Check sheet for the modelled part. Datum: model origin and axes. Units: mm. Coordinates: 2 decimals unless noted, no trailing zeros. Order: outer loops, then holes, each group sorted by start corner. A loop starts at its lowest first (then second) coordinate and runs counter-clockwise, first axis right, second up.
1. Draft check along Y on faces 1 (the cylindrical face through (21.09, -41.027, 1.29)), 2 (the cylindrical face through (-16.44, 33.2, 1.29)), 3 (the flat face through (0, 1, 2)), 4 (the cylindrical face through (24.837, 48.709, 1.29)). Enter one of: released by +Y, released by -Y, zero draft, split by the parting line, or undercut.
2. Thickness scan on line 1 (X direction, y = 10, z = 1.05); line 2 (Y direction, x = 21.5, z = 1.65). Record the ranges inside material, lowest first.
3. Cross-section at A-A (y = -10.5). Enter the section's corners in (x, z).
4. Gauge pin test, flat ends, axial feed: pin 1 Ø0.7 at (x, z) = (6, 1) entering from +Y; pin 2 Ø0.7 at (x, z) = (-12, 1.5) entering from +Y; pin 3 Ø1.1 at (x, z) = (8.5, 1) entering from +Y; pin 4 Ø2.5 at (x, y) = (15.25, 3.61) entering from +Z. Record the tip position at first contact, or that the pin passes through.
```python
from build123d import *

# Parameters (mm, degrees)
F0_R     = 3.15
F0_W     = 5
F0_H     = 2.5
F0_W_2   = 30
F0_H_2   = 13
F0_R_2   = 1.5
F1_DEPTH = 2
F2_SIZE  = 0.6
F3_SIZE  = 1


with BuildPart() as f1:
    # F0 (on Top) → F1 (new body)
    with BuildSketch(Plane.XY):
        with BuildLine():
            ThreePointArc((19.649657, 49.48842), (0, 46.17961), (-19.649657, 49.48842))
            ThreePointArc((-19.649657, 49.48842), (-24.776283, 48.753093), (-27.15, 44.15))
            Line((-27.15, 44.15), (-27.15, -44.15))
            ThreePointArc((-27.15, -44.15), (-24.776283, -48.753093), (-19.649657, -49.48842))
            ThreePointArc((-19.649657, -49.48842), (0, -46.17961), (19.649657, -49.48842))
            ThreePointArc((19.649657, -49.48842), (24.776283, -48.753093), (27.15, -44.15))
            Line((27.15, -44.15), (27.15, 44.15))
            ThreePointArc((27.15, 44.15), (24.776283, 48.753093), (19.649657, 49.48842))
        make_face()
        with Locations((-21.5, -44.15)):
            Circle(F0_R, mode=Mode.SUBTRACT)
        with Locations((-12.882352, -38.913459)):
            Rectangle(F0_W, F0_H, mode=Mode.SUBTRACT)
        with Locations((-12.882352, -5.600822)):
            Rectangle(F0_W, F0_H, mode=Mode.SUBTRACT)
        with Locations((7.687139, -38.913459)):
            Rectangle(F0_W, F0_H, mode=Mode.SUBTRACT)
        with Locations((21.5, -44.15)):
            Circle(F0_R, mode=Mode.SUBTRACT)
        with Locations((0, -22.107908)):
            Rectangle(F0_W_2, F0_H_2, mode=Mode.SUBTRACT)
        with Locations((7.687139, -5.600822)):
            Rectangle(F0_W, F0_H, mode=Mode.SUBTRACT)
        with BuildLine():
            ThreePointArc((-22.65, -34), (-22.942893, -34.707107), (-23.65, -35))
            ThreePointArc((-23.65, -35), (-24.357107, -34.707107), (-24.65, -34))
            Line((-24.65, -34), (-24.65, 34))
            ThreePointArc((-24.65, 34), (-24.357107, 34.707107), (-23.65, 35))
            ThreePointArc((-23.65, 35), (-22.942893, 34.707107), (-22.65, 34))
            Line((-22.65, 34), (-22.65, -34))
        make_face(mode=Mode.SUBTRACT)
        with Locations((-15.25, 3.611581)):
            Circle(F0_R_2, mode=Mode.SUBTRACT)
        with Locations((-6.775575, 7.31866)):
            Rectangle(F0_W, F0_H, mode=Mode.SUBTRACT)
        with Locations((-15.25, 34.111581)):
            Circle(F0_R_2, mode=Mode.SUBTRACT)
        with Locations((-21.5, 44.15)):
            Circle(F0_R, mode=Mode.SUBTRACT)
        with Locations((-6.775575, 36.897157)):
            Rectangle(F0_W, F0_H, mode=Mode.SUBTRACT)
        with Locations((6.775575, 7.31866)):
            Rectangle(F0_W, F0_H, mode=Mode.SUBTRACT)
        with Locations((0, 22.107908)):
            Rectangle(F0_W_2, F0_H_2, mode=Mode.SUBTRACT)
        with Locations((15.25, 3.611581)):
            Circle(F0_R_2, mode=Mode.SUBTRACT)
        with BuildLine():
            Line((22.65, -34), (22.65, 34))
            ThreePointArc((22.65, 34), (22.942893, 34.707107), (23.65, 35))
            ThreePointArc((23.65, 35), (24.357107, 34.707107), (24.65, 34))
            Line((24.65, 34), (24.65, -34))
            ThreePointArc((24.65, -34), (24.357107, -34.707107), (23.65, -35))
            ThreePointArc((23.65, -35), (22.942893, -34.707107), (22.65, -34))
        make_face(mode=Mode.SUBTRACT)
        with Locations((6.775575, 36.897157)):
            Rectangle(F0_W, F0_H, mode=Mode.SUBTRACT)
        with Locations((15.25, 34.111581)):
            Circle(F0_R_2, mode=Mode.SUBTRACT)
        with Locations((21.5, 44.15)):
            Circle(F0_R, mode=Mode.SUBTRACT)
    extrude(amount=F1_DEPTH)

    # F2
    f2_edges = [f1.edges().sort_by_distance(p)[0] for p in [
        (27.15, 0, 0),
        (18.35, -44.15, 0),
        (-24.65, -44.15, 0),
        (-15.382352, -38.913459, 0),
        (-12.882352, -37.663459, 0),
        (-10.382352, -38.913459, 0),
        (-12.882352, -40.163459, 0),
        (5.187139, -38.913459, 0),
        (7.687139, -37.663459, 0),
        (10.187139, -38.913459, 0),
        (7.687139, -40.163459, 0),
        (0, -28.607908, 0),
        (15, -22.107908, 0),
        (0, -15.607908, 0),
        (-15, -22.107908, 0),
        (-15.382352, -5.600822, 0),
        (-12.882352, -6.850822, 0),
        (-10.382352, -5.600822, 0),
        (-12.882352, -4.350822, 0),
        (5.187139, -5.600822, 0),
        (7.687139, -4.350822, 0),
        (7.687139, -6.850822, 0),
        (10.187139, -5.600822, 0),
        (13.75, 3.611581, 0),
        (-16.75, 3.611581, 0),
        (9.275575, 7.31866, 0),
        (6.775575, 8.56866, 0),
        (6.775575, 6.06866, 0),
        (4.275575, 7.31866, 0),
        (-4.275575, 7.31866, 0),
        (-6.775575, 8.56866, 0),
        (-6.775575, 6.06866, 0),
        (-9.275575, 7.31866, 0),
        (0, 15.607908, 0),
        (15, 22.107908, 0),
        (0, 28.607908, 0),
        (-15, 22.107908, 0),
        (13.75, 34.111581, 0),
        (9.275575, 36.897157, 0),
        (6.775575, 35.647157, 0),
        (6.775575, 38.147157, 0),
        (4.275575, 36.897157, 0),
        (-4.275575, 36.897157, 0),
        (-6.775575, 38.147157, 0),
        (-6.775575, 35.647157, 0),
        (-9.275575, 36.897157, 0),
        (18.35, 44.15, 0),
        (-24.65, 44.15, 0),
        (-16.75, 34.111581, 0),
        (22.65, 0, 2),
        (-22.65, 0, 2),
    ]]
    chamfer(f2_edges, length=F2_SIZE)

    # F3
    f3_edges = [f1.edges().sort_by_distance(p)[0] for p in [
        (22.65, 0, 0),
        (-22.65, 0, 0),
    ]]
    chamfer(f3_edges, length=F3_SIZE)


solid = f1.part
```
Data:
1. face 1: undercut
1. face 2: undercut
1. face 3: zero draft
1. face 4: released by +Y
2. line 1: x = -27.15 to -24.65, -22.65 to 22.65, 24.65 to 27.15
2. line 2: y = -49.8 to -47.3, -41 to 41, 47.3 to 49.8
3. outline: (-27.15, 0.6) - (-26.55, 0) - (-25.65, 0) - (-24.65, 1) - (-24.65, 1.4) - (-25.25, 2) - (-27.15, 2) - close; (-22.65, 1) - (-21.65, 0) - (21.65, 0) - (22.65, 1) - (22.65, 1.4) - (22.05, 2) - (-22.05, 2) - (-22.65, 1.4) - close; (24.65, 1) - (25.65, 0) - (26.55, 0) - (27.15, 0.6) - (27.15, 2) - (25.25, 2) - (24.65, 1.4) - close
4. pin 1: stops at y = 46.52
4. pin 2: stops at y = 47.46
4. pin 3: stops at y = 46.87
4. pin 4: passes through
